Model file for the job. Use its own axes, mm. A direction names the side the tool comes from. Round coordinates to 2 decimals unless told otherwise and drop trailing zeros. Loops run counter-clockwise (first coordinate to the right, second up) from the corner with the lowest first, then second, coordinate; pieces in that order, holes last.
from build123d import *

# Parameters (mm, degrees)
CUT_EXTRUDE_1316_DEPTH = 9
CUT_EXTRUDE_1657_DEPTH = 2
SKETCH_3_R             = 8.75
CUT_EXTRUDE_1713_DEPTH = 7
SKETCH_1963_R          = 2.25
CUT_EXTRUDE_2333_DEPTH = 51.545474575


with BuildPart() as part:
    # Sketch 1 → Revolve 1 (revolve)
    with BuildSketch(Plane.XY, mode=Mode.PRIVATE) as revolve_1_sk:
        Polygon((0, 26), (30.65, 26), (30.65, 0), (18.65, 0), (18.65, 7), (17.15, 7), (17.15, 13.5), (3.65, 13.5), (3.65, 17), (0, 17), align=None)
    revolve(revolve_1_sk.sketch.rotate(Axis((0, 0, 0), (0, 1, 0)), 90), axis=Axis((0, 0, 0), (0, 1, 0)))

    # Sketch 667 → Cut-Extrude 1316 (cut)
    with BuildSketch(Plane(origin=(0, 26, 0), x_dir=(1, 0, 0), z_dir=(0, 1, 0))):
        with BuildLine():
            Line((5.65, -6.681317235), (5.65, 6.681317235))
            ThreePointArc((5.65, 6.681317235), (0.957048309, 8.697503006), (-4.062019202, 7.75))
            Line((-4.062019202, 7.75), (-4.062019202, -7.75))
            ThreePointArc((-4.062019202, -7.75), (0.957048309, -8.697503006), (5.65, -6.681317235))
        make_face()
        with BuildLine():
            Line((-4.062019202, -7.75), (-4.062019202, 7.75))
            ThreePointArc((-4.062019202, 7.75), (-4.885319842, 7.259211392), (-5.65, 6.681317235))
            Line((-5.65, 6.681317235), (-5.65, -6.681317235))
            ThreePointArc((-5.65, -6.681317235), (-4.885319842, -7.259211392), (-4.062019202, -7.75))
        make_face()
    extrude(amount=-CUT_EXTRUDE_1316_DEPTH, mode=Mode.SUBTRACT)

    # Sketch 1370 → Cut-Extrude 1657 (cut)
    with BuildSketch(Plane(origin=(0, 17, 0), x_dir=(1, 0, 0), z_dir=(0, 1, 0))):
        with BuildLine():
            Line((-0.92, -7.2), (0.92, -7.2))
            ThreePointArc((0.92, -7.2), (1.330121933, -7.369878067), (1.5, -7.78))
            Line((1.5, -7.78), (1.5, -8.082233602))
            ThreePointArc((1.5, -8.082233602), (1.341523495, -8.496233679), (0.947109471, -8.6985909))
            ThreePointArc((0.947109471, -8.6985909), (0, -8.75), (-0.947109471, -8.6985909))
            ThreePointArc((-0.947109471, -8.6985909), (-1.341523495, -8.496233679), (-1.5, -8.082233602))
            Line((-1.5, -8.082233602), (-1.5, -7.78))
            ThreePointArc((-1.5, -7.78), (-1.330121933, -7.369878067), (-0.92, -7.2))
        make_face()
    extrude(amount=-CUT_EXTRUDE_1657_DEPTH, mode=Mode.SUBTRACT)

    # Sketch 3 → Cut-Extrude 1713 (cut)
    with BuildSketch(Plane(origin=(0, 26, 0), x_dir=(1, 0, 0), z_dir=(0, 1, 0))):
        Circle(SKETCH_3_R)
        with BuildLine():
            Line((5.65, 6.681317235), (5.65, -6.681317235))
            ThreePointArc((5.65, -6.681317235), (0, -8.75), (-5.65, -6.681317235))
            Line((-5.65, -6.681317235), (-5.65, 6.681317235))
            ThreePointArc((-5.65, 6.681317235), (0, 8.75), (5.65, 6.681317235))
        make_face()
        with BuildLine():
            Line((-17.062019202, 7.75), (-30.620254734, 1.35))
            ThreePointArc((-30.620254734, 1.35), (-30.65, 0), (-30.620254734, -1.35))
            Line((-30.620254734, -1.35), (-17.062019202, -7.75))
            Line((-17.062019202, -7.75), (-4.062019202, -7.75))
            Line((-4.062019202, -7.75), (-4.062019202, 7.75))
            Line((-4.062019202, 7.75), (-17.062019202, 7.75))
        make_face()
    extrude(amount=-CUT_EXTRUDE_1713_DEPTH, mode=Mode.SUBTRACT)

    # Sketch 1963 → Cut-Extrude 2333 (cut, through all)
    with BuildSketch(Plane(origin=(0, 26, 0), x_dir=(1, 0, 0), z_dir=(0, 1, 0))):
        with Locations(Location((24.65, 0, 0), (0, 0, 270))):
            Circle(SKETCH_1963_R)
        with Locations(Location((-12.325, -21.347526203, 0), (0, 0, 270))):
            Circle(SKETCH_1963_R)
        with Locations(Location((-12.325, 21.347526203, 0), (0, 0, 270))):
            Circle(SKETCH_1963_R)
    extrude(amount=-CUT_EXTRUDE_2333_DEPTH, mode=Mode.SUBTRACT)


solid = part.part
Q1. Tool access for faces 1 (the face through (-11.65, 13.18, -19.2)), 2 (the face through (-4, 13.5, 0)), 3 (the face through (-5.65, 18, 0)): list every direction of +Z, -Z, +X, -X, +Y, -Y with a clear straight run to the whole face (end or side of a thin tool).
Q2. Slice it at D-D on y = 18. Give the cut face in (x, z) (3 decimals), plus the area to 3 significant figures.
Q3. Slice it at C-C on z = 21. Give the cut face in (x, y).
Q4. Slice it at A-A on x = 0. Give the cut face in (y, z).
Q5. Probe line 1 (X direction, y = 6, z = 0); line 2 (X direction, y = 15.7, z = 0); line 3 (Y direction, x = -21.5, z = 1.5). List the from-to ranges inside material, lowest first.
Q6. Slice it at B-B on z = 0. Give the cut face in (x, y).
Q7. Pull direction X, two halves, no side cores. Call faces 4 (the face through (20, 0, 0)), 5 (the face through (-30.39, 12.82, 3.99)), 6 (the face through (-10.804, 13.182, 19.689)): pulls with the +X half, pulls with the -X half, needs draft (parallel to the pull), parting line crosses it, or undercut.
Q8. Flat gauge pins, fed straight in: P1, Ø1.5, axis at x = -11.5, y = 12, coming from the -Z side; P2, Ø0.6, axis at y = 18, z = -1.5, coming from the +X side; P3, Ø5.5, axis at x = -9, y = 23.5, coming from the -Z side; P4, Ø4, axis at x = 16.5, z = -14, coming from the -Y side. Where does each tip first touch, or does it go through?
Reply:
1. face 1: +Y, -Y
1. face 2: -Y
1. face 3: +Y
2. outline: circle Ø61.3 at (0, 0); hole circle Ø4.5 at (-12.325, -21.348); hole circle Ø4.5 at (-12.325, 21.348); hole (-5.65, -6.681) arc R8.75 ccw to (5.65, -6.681) - (5.65, 6.681) arc R8.75 ccw to (-5.65, 6.681) - close; hole circle Ø4.5 at (24.65, 0)
2. area: 2,720 mm2
3. outline: (-22.33, 0) - (-14.55, 0) - (-14.55, 26) - (-22.33, 26) - close; (-10.1, 0) - (22.33, 0) - (22.33, 26) - (-10.1, 26) - close
4. outline: (0, -30.65) - (26, -30.65) - (26, -8.75) - (17, -8.75) - (17, -3.65) - (13.5, -3.65) - (13.5, -17.15) - (7, -17.15) - (7, -18.65) - (0, -18.65) - close; (0, 18.65) - (7, 18.65) - (7, 17.15) - (13.5, 17.15) - (13.5, 3.65) - (17, 3.65) - (17, 7.2) - (15, 7.2) - (15, 8.75) - (26, 8.75) - (26, 30.65) - (0, 30.65) - close
5. line 1: x = -30.65 to -18.65, 18.65 to 22.4, 26.9 to 30.65
5. line 2: x = -30.65 to -3.65, 3.65 to 22.4, 26.9 to 30.65
5. line 3: y = 0 to 19
6. outline: (-30.65, 0) - (-18.65, 0) - (-18.65, 7) - (-17.15, 7) - (-17.15, 13.5) - (-3.65, 13.5) - (-3.65, 17) - (-5.65, 17) - (-5.65, 19) - (-30.65, 19) - close; (3.65, 13.5) - (17.15, 13.5) - (17.15, 7) - (18.65, 7) - (18.65, 0) - (22.4, 0) - (22.4, 26) - (8.75, 26) - (8.75, 19) - (5.65, 19) - (5.65, 17) - (3.65, 17) - close; (26.9, 0) - (30.65, 0) - (30.65, 26) - (26.9, 26) - close
7. face 4: needs draft
7. face 5: parting line crosses it
7. face 6: undercut
8. P1: stops at z = -28.7
8. P2: stops at x = 30.63
8. P3: stops at z = -30.01
8. P4: stops at y = 0
